Drawing for the job (mm, zero at the part's lowest x, y, z). A direction names the side the tool comes from. Give positions to 0.01 mm unless a question says otherwise; leave off trailing zeros. Loops run counter-clockwise (first coordinate to the right, second up) from the corner with the lowest first, then second, coordinate; pieces in that order, holes last. Notation, with made-up numbers: (35.25, 65) -> (54.25, 65) arc R20 ccw to (54.25, 73) -> close; hole circle Ø9 at (-23, 35). An arc over 180 degrees is marked (long way). Write item = value, one per line.
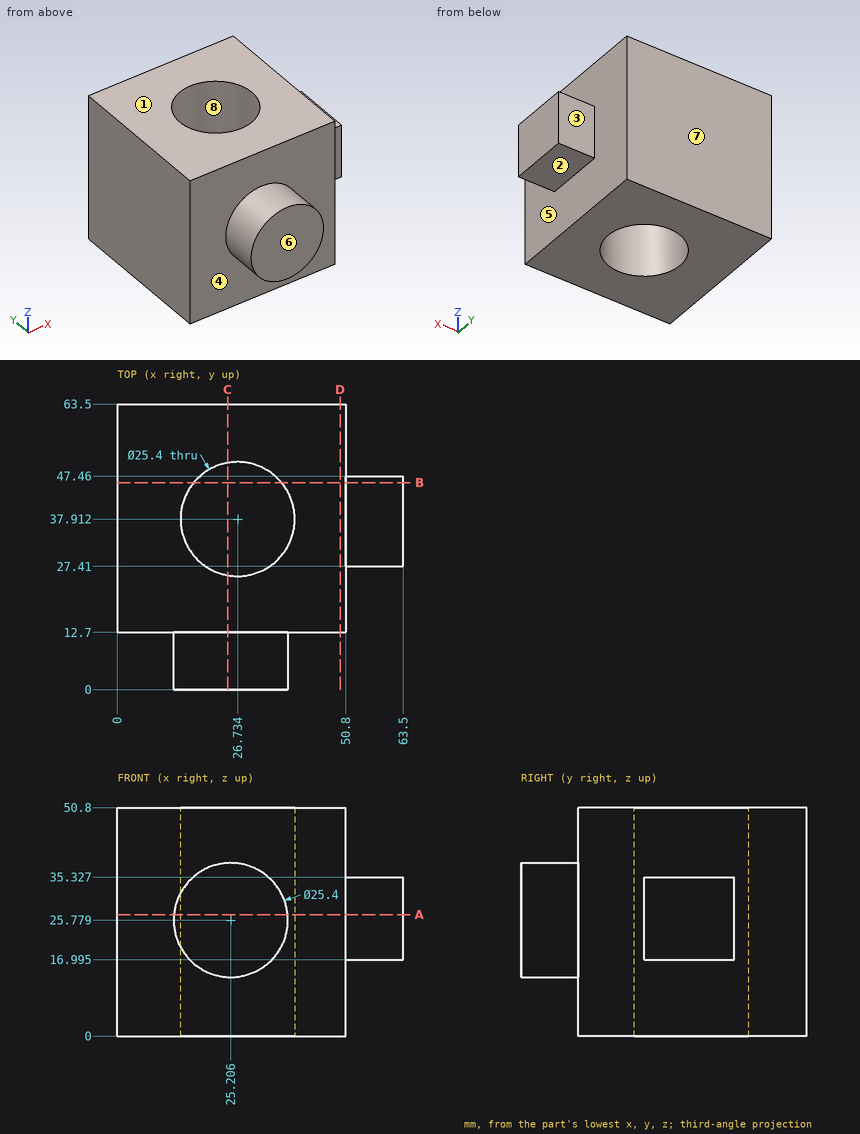
1) Slice it at A-A, the plane z = 27. List the corners of the cut face in (x, y) (1 decimal).
Resolved:
outline = (0, 12.7) -> (12.6, 12.7) -> (12.6, 0) -> (37.8, 0) -> (37.8, 12.7) -> (50.8, 12.7) -> (50.8, 27.4) -> (63.5, 27.4) -> (63.5, 47.5) -> (50.8, 47.5) -> (50.8, 63.5) -> (0, 63.5) -> close; hole circle Ø25.4 at (26.7, 37.9)
2) Slice it at D-D, the plane x = 49.5. List the corners of the cut face in (y, z).
Resolved:
outline = (12.7, 0) -> (63.5, 0) -> (63.5, 50.8) -> (12.7, 50.8) -> close
3) Slice it at C-C, the plane x = 24.5. List the corners of the cut face in (y, z), and give its area (3 significant figures).
Resolved:
outline = (0, 13.1) -> (12.7, 13.1) -> (12.7, 0) -> (25.41, 0) -> (25.41, 50.8) -> (12.7, 50.8) -> (12.7, 38.46) -> (0, 38.46) -> close; (50.41, 0) -> (63.5, 0) -> (63.5, 50.8) -> (50.41, 50.8) -> close
area = 1,630 mm²
4) Slice it at B-B, the plane y = 46. List the corners of the cut face in (x, z) (1 decimal).
Resolved:
outline = (0, 0) -> (16.9, 0) -> (16.9, 50.8) -> (0, 50.8) -> close; (36.5, 0) -> (50.8, 0) -> (50.8, 17) -> (63.5, 17) -> (63.5, 35.3) -> (50.8, 35.3) -> (50.8, 50.8) -> (36.5, 50.8) -> close
5) Pull direction Y, two halves, no side cores. Call the marked faces 5, 6, 7 and 8: pulls with the +Y half, pulls with the -Y half, needs draft (parallel to the pull), parting line crosses it, or undercut.
Resolved:
face_5 = needs draft
face_6 = pulls with the -Y half
face_7 = pulls with the +Y half
face_8 = undercut
6) Drop flat-ended pins along their axis: P1, Ø5, axis at x = 18, y = 17.5, coming from the -Z side; P2, Ø10, axis at x = 58.5, y = 39.5, coming from the +Z side; P3, Ø23, axis at x = 26.73, y = 37.91, coming from the +Z side; P4, Ø4, axis at x = 55.5, y = 39.5, coming from the -Z side (3 decimals). Give the stop position or say it passes through.
Resolved:
P1 = 0
P2 = 35.33
P3 = through
P4 = 16.995
7) Drill centre lines: line 1 along X through (y, z) = (13, 14.5); line 2 along Z through (x, y) = (52, 43) (1 decimal); line 3 along Y through (x, z) = (6.5, 45). Where is each one in solid material? Low to high. Write a range as [from, to].
Resolved:
line_1 = [0, 50.8]
line_2 = [17, 35.3]
line_3 = [12.7, 63.5]
8) Which spindle directions (+Z, -Z, +X, -X, +Y, -Y) get a long thin tool onto all of the face, cutting with end or side? Do the marked faces 1, 2, 3 and 4. Say none if no direction does.
Resolved:
face_1 = +Z, +X, -X, +Y, -Y
face_2 = -Z, +X, +Y, -Y
face_3 = +Z, -Z, +X, +Y
face_4 = -Y
